```python
from build123d import *

# Parameters (mm, degrees)
SKETCH1_W           = 310
SKETCH1_H           = 85
BOSS_EXTRUDE1_DEPTH = 10
SKETCH2_W           = 310
SKETCH2_H           = 100
BOSS_EXTRUDE2_DEPTH = 10
SKETCH3_R           = 40
CUT_EXTRUDE1_DEPTH  = 10
SKETCH4_R           = 40
BOSS_EXTRUDE3_DEPTH = 20


with BuildPart() as part:
    # Sketch1 → Boss-Extrude1 (new body)
    with BuildSketch(Plane.XY):
        with Locations((-95, 42.5)):
            Rectangle(SKETCH1_W, SKETCH1_H)
        with BuildLine():
            Line((-250, 85), (0, 85))
            Line((0, 85), (0, 165))
            add(Edge.make_bspline(
                [(-250, 85), (-173.352632869, 120.304599368), (-81.564360867, 181.904903874), (0, 165)],
                knots=[0, 0, 0, 0, 0.796760971, 0.796760971, 0.796760971, 0.796760971], degree=3))
        make_face()
        with BuildLine():
            Line((0, 85), (60, 85))
            Line((60, 85), (60, 135))
            add(Edge.make_bspline(
                [(0, 165), (20.805564215, 160.687870789), (40.945893284, 151.267674504), (60, 135)],
                knots=[0.796760971, 0.796760971, 0.796760971, 0.796760971, 1, 1, 1, 1], degree=3))
            Line((0, 165), (0, 85))
        make_face()
    boss_extrude1 = extrude(amount=-BOSS_EXTRUDE1_DEPTH)

    # Sketch2 → Boss-Extrude2 (add)
    with BuildSketch(Plane(origin=(0, 0, 0), x_dir=(1, 0, 0), z_dir=(0, 1, 0))):
        with Locations((-95, 60)):
            Rectangle(SKETCH2_W, SKETCH2_H)
    extrude(amount=BOSS_EXTRUDE2_DEPTH)

    # Sketch3 → Cut-Extrude1 (cut)
    with BuildSketch(Plane.XY):
        with Locations((0, 85)):
            Circle(SKETCH3_R)
    cut_extrude1 = extrude(amount=-CUT_EXTRUDE1_DEPTH, mode=Mode.SUBTRACT)

    # Mirror1: Boss-Extrude1, Cut-Extrude1 across plane
    add(boss_extrude1.mirror(Plane(origin=(0, 0, -55), x_dir=(1, 0, 0), z_dir=(0, 0, -1))))
    add(cut_extrude1.mirror(Plane(origin=(0, 0, -55), x_dir=(1, 0, 0), z_dir=(0, 0, -1))), mode=Mode.SUBTRACT)

    # Sketch4 → Boss-Extrude3 (add)
    with BuildSketch(Plane.XZ):
        with Locations(Location((0, -55, 0), (0, 0, 180))):
            Circle(SKETCH4_R)
    extrude(amount=BOSS_EXTRUDE3_DEPTH)


solid = part.part
```
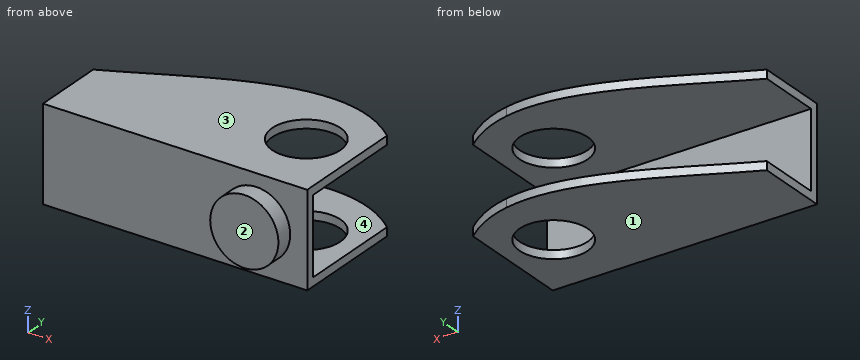
Here's how the part is built. I have some questions about the finished solid (model axes, mm). Face numbers are marked on the shaded views. Give positions to 0.01 mm unless a question says otherwise; leave off trailing zeros. Order: outer loops, then holes, each group sorted by start corner. A loop starts at its lowest first (then second) coordinate and runs counter-clockwise, first axis right, second up. Notation, with made-up numbers: M 5.5,-2 L 51.5,-2 A4 cw 51.5,5 Z; hole C -37.5,-22.75 d5. An arc over 180 degrees is marked long. Use a Markdown table: item, result. Add a question column.
1. Suppose I cut it at C-C (y = 75). List the corners of the cut face in (x, z) for me, and give its area (3 significant figures).
2. Suppose I cut it at D-D (z = -19.5). List the corners of the cut face in (x, y) for me.
3. I need wall thicknesses on probe 1 along Y at (x, z) = (0, -106); probe 2 along Z at (x, y) = (-7.5, 33); probe 3 along Y at (x, z) = (-190, -26.5). Which ranges of each line are inside material? Lowest first, please. Write a range as from..to.
4. Suppose I cut it at A-A (z = -55). List the corners of the cut face in (x, y) for me, and give its area (3 significant figures).
5. For pin 1 Ø3 at (x, z) = (-51, -81) entering from -Y; pin 2 Ø1 at (x, z) = (-80, -38) entering from +Y, each with a flat end and sliding along its axis, tell me the tip position at first contact or that it passes through.
6. Suppose I cut it at B-B (y = 55). List the corners of the cut face in (x, z) for me, and give its area (3 significant figures).
7. If we mould it in two halves opening along Z, with no side actions, what happens to the marked faces 1, 2, 3 and 4? For each: +Z half, -Z half, draft (parallel to the pull), parting line (faces both ways), or undercut.
Results list:
| question | item | result |
|---|---|---|
| 1 | outline | M -250,-110 L -38.73,-110 L -38.73,-100 L -250,-100 Z; M -250,-10 L -38.73,-10 L -38.73,0 L -250,0 Z; M 38.73,-110 L 60,-110 L 60,-100 L 38.73,-100 Z; M 38.73,-10 L 60,-10 L 60,0 L 38.73,0 Z |
| 1 | area | 4,650 mm² |
| 2 | outline | M -250,0 L -18.43,0 L -18.43,-20 L 18.43,-20 L 18.43,0 L 60,0 L 60,10 L -250,10 Z |
| 3 | probe 1 | y = 0..45, 125..165 |
| 3 | probe 2 | z = -110..-100, -10..0 |
| 3 | probe 3 | y = 0..10 |
| 4 | outline | M -250,0 L -40,0 L -40,-20 L 40,-20 L 40,0 L 60,0 L 60,10 L -250,10 Z |
| 4 | area | 4,700 mm² |
| 5 | pin 1 | stops at y = 0 |
| 5 | pin 2 | stops at y = 10 |
| 6 | outline | M -250,-110 L -26.46,-110 L -26.46,-100 L -250,-100 Z; M -250,-10 L -26.46,-10 L -26.46,0 L -250,0 Z; M 26.46,-110 L 60,-110 L 60,-100 L 26.46,-100 Z; M 26.46,-10 L 60,-10 L 60,0 L 26.46,0 Z |
| 6 | area | 5,140 mm² |
| 7 | face 1 | -Z half |
| 7 | face 2 | draft |
| 7 | face 3 | +Z half |
| 7 | face 4 | undercut |
